Here's how the part is built. I have some questions about the finished solid (model axes, mm). A direction names the side the tool comes from. Round coordinates to 2 decimals unless told otherwise and drop trailing zeros. Loops run counter-clockwise (first coordinate to the right, second up) from the corner with the lowest first, then second, coordinate; pieces in that order, holes last. Notation, with made-up numbers: (-7.75, 16) -> (21.25, 16) arc R12 cw to (21.25, 39) -> close; hole circle Ø9 at (26, 86). An arc over 180 degrees is marked (long way). Use one line per item in the form item = value. Start each with the question number.
Item 1: If we section it at A-A (x = 0): Write out the boundary of the cut face in (y, z).
Item 2: I'm going to push flat-ended pins straight in: pin 1 Ø3 at (x, z) = (37.5, -22.5) entering from -Y; pin 2 Ø2 at (y, z) = (1.5, -25) entering from -X. Where does each tip first touch, or does it pass through?
Item 3: If I drill on L1, parallel to Z at x = -40.5, y = 2.35; L2, parallel to X at y = 4.25, z = -1, over which ranges is the centre line in solid material (lowest first)? Write a range as [from, to].
Item 4: Thinking about a two-plate mould opening in X: for faces 1 (the face through (-47.5, 2, 22)), 2 (the face through (-40.934, 2.535, -38.548)), 3 (the face through (40.066, 2.535, -38.548)), 4 (the face through (-1, 2, 47.5)), which applies, released by +X, released by -X, zero draft, split by the parting line, or undercut?
Item 5: If we section it at B-B (y = 2.85): Write out the boundary of the cut face in (x, z), then the cut area to 3 significant figures.
Item 6: If we section it at C-C (z = -7): Write out the boundary of the cut face in (x, y).
Item 7: For faces 5 (the face through (-48.979, 2.465, -1.423)), 6 (the face through (-48.98, 2.53, 1.46)), 7 (the face through (47.5, 2, 1)), which set-ups out of +Z, -Z, +X, -X, +Y, -Y let a thin tool reach every point of the face, with its end or its side?
```python
from build123d import *

# Parameters (mm, degrees)
SKETCH1_W             = 95
SKETCH1_H             = 95
SKETCH1_W_2           = 81
SKETCH1_H_2           = 81
SKETCH1_R             = 40.1
BOSS_EXTRUDE1_DEPTH   = 5
F_4_0MM_DOWEL_HOLE1_D = 4
BOSS_EXTRUDE2_DEPTH   = 3
FILLET1_R             = 5


with BuildPart() as part:
    # Sketch1 → Boss-Extrude1 (new body)
    # profile 1 of 2: a face of its own
    with BuildSketch(Plane(origin=(0, 0, 0), x_dir=(1, 0, 0), z_dir=(0, 1, 0))):
        Rectangle(SKETCH1_W, SKETCH1_H)
        Rectangle(SKETCH1_W_2, SKETCH1_H_2, mode=Mode.SUBTRACT)
    # profile 2 of 2: a face of its own
    with BuildSketch(Plane(origin=(0, 0, 0), x_dir=(1, 0, 0), z_dir=(0, 1, 0))):
        Rectangle(SKETCH1_W_2, SKETCH1_H_2)
        with Locations(Location((0, 0, 0), (0, 0, 270))):
            Circle(SKETCH1_R, mode=Mode.SUBTRACT)
    extrude(amount=BOSS_EXTRUDE1_DEPTH)

    # Ø4.0mm Dowel Hole1 (through all)
    with Locations(Plane(origin=(0, 0, 0), x_dir=(-1, 0, 0), z_dir=(0, -1, 0))):
        with Locations((40.5, -40.5), (-40.5, -40.5), (-40.5, 40.5), (40.5, 40.5)):
            Hole(F_4_0MM_DOWEL_HOLE1_D / 2)

    # Sketch5 → Boss-Extrude2 (add)
    with BuildSketch(Plane.ZY.offset(47.5)):
        Polygon((0, 0), (-2.886751346, 5), (2.886751346, 5), align=None)
    extrude(amount=BOSS_EXTRUDE2_DEPTH)

    # Fillet1
    fillet1_edges = [part.edges().sort_by_distance(p)[0] for p in [
        (-47.5, 2.5, 47.5),
        (-47.5, 2.5, -47.5),
        (47.5, 2.5, -47.5),
        (47.5, 2.5, 47.5),
    ]]
    fillet(fillet1_edges, radius=FILLET1_R)


solid = part.part
```
Values found:
q1.outline = (0, -47.5) -> (5, -47.5) -> (5, -40.1) -> (0, -40.1) -> close; (0, 40.1) -> (5, 40.1) -> (5, 47.5) -> (0, 47.5) -> close
q2.pin_1 = 0
q2.pin_2 = -47.5
q3.L1 = [-47.5, -42.5], [-38.5, 38.5], [42.5, 47.5]
q3.L2 = [-50.5, -40.09], [40.09, 47.5]
q4.face_1 = released by -X
q4.face_2 = undercut
q4.face_3 = undercut
q4.face_4 = zero draft
q5.outline = (-50.5, -1.65) -> (-47.5, -1.65) -> (-47.5, -42.5) arc R5 ccw to (-42.5, -47.5) -> (42.5, -47.5) arc R5 ccw to (47.5, -42.5) -> (47.5, 42.5) arc R5 ccw to (42.5, 47.5) -> (-42.5, 47.5) arc R5 ccw to (-47.5, 42.5) -> (-47.5, 1.65) -> (-50.5, 1.65) -> close; hole circle Ø4 at (-40.5, -40.5); hole circle Ø4 at (-40.5, 40.5); hole circle Ø80.2 at (0, 0); hole circle Ø4 at (40.5, -40.5); hole circle Ø4 at (40.5, 40.5)
q5.area = 3,910 mm2
q6.outline = (-47.5, 0) -> (-39.48, 0) -> (-39.48, 5) -> (-47.5, 5) -> close; (39.48, 0) -> (47.5, 0) -> (47.5, 5) -> (39.48, 5) -> close
q7.face_5 = -Z, -X, -Y
q7.face_6 = +Z, -X, -Y
q7.face_7 = +Z, -Z, +X, +Y, -Y
